Part model, mm, in its own coordinate system. Give positions to 0.01 mm unless a question says otherwise; leave off trailing zeros. Order: outer loops, then holes, each group sorted by start corner. A loop starts at its lowest first (then second) coordinate and runs counter-clockwise, first axis right, second up.
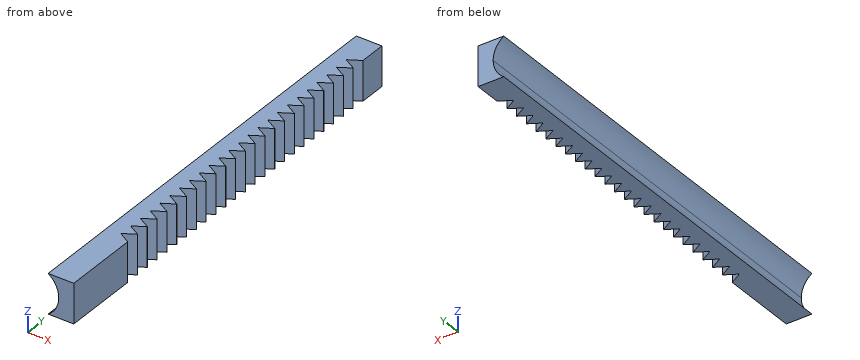
from build123d import *

# Parameters (mm, degrees)
BOSS_EXTRUDE1_DEPTH = 550
CUT_EXTRUDE1_DEPTH  = 73
BOSS_EXTRUDE2_DEPTH = 550


with BuildPart() as part:
    # Sketch1 → Boss-Extrude1 (new body)
    with BuildSketch(Plane(origin=(0, 0, 0), x_dir=(1, 0, 0), z_dir=(0, 1, 0))):
        with BuildLine():
            Line((43.301270189, -25), (69, -25))
            Line((69, -25), (69, 25))
            Line((69, 25), (43.301270189, 25))
            ThreePointArc((43.301270189, 25), (50, 0), (43.301270189, -25))
        make_face()
    extrude(amount=BOSS_EXTRUDE1_DEPTH)

    # Sketch2 → Cut-Extrude1 (cut)
    with BuildSketch(Plane.XY.offset(25)):
        Polygon((54, 489.993192311), (76.5, 477.002811254), (76.5, 502.983573367), align=None)
        Polygon((54, 507.493192311), (76.5, 494.502811254), (76.5, 520.483573367), align=None)
        Polygon((54, 472.493192311), (76.5, 459.502811254), (76.5, 485.483573367), align=None)
        Polygon((54, 454.993192311), (76.5, 442.002811254), (76.5, 467.983573367), align=None)
        Polygon((54, 437.493192311), (76.5, 424.502811254), (76.5, 450.483573367), align=None)
        Polygon((54, 419.993192311), (76.5, 407.002811254), (76.5, 432.983573367), align=None)
        Polygon((54, 402.493192311), (76.5, 389.502811254), (76.5, 415.483573367), align=None)
        Polygon((54, 384.993192311), (76.5, 372.002811254), (76.5, 397.983573367), align=None)
        Polygon((54, 367.493192311), (76.5, 354.502811254), (76.5, 380.483573367), align=None)
        Polygon((54, 349.993192311), (76.5, 337.002811254), (76.5, 362.983573367), align=None)
        Polygon((54, 332.493192311), (76.5, 319.502811254), (76.5, 345.483573367), align=None)
        Polygon((54, 314.993192311), (76.5, 302.002811254), (76.5, 327.983573367), align=None)
        Polygon((54, 297.493192311), (76.5, 284.502811254), (76.5, 310.483573367), align=None)
        Polygon((54, 279.993192311), (76.5, 267.002811254), (76.5, 292.983573367), align=None)
        Polygon((54, 262.493192311), (76.5, 249.502811254), (76.5, 275.483573367), align=None)
        Polygon((54, 244.993192311), (76.5, 232.002811254), (76.5, 257.983573367), align=None)
        Polygon((54, 227.493192311), (76.5, 214.502811254), (76.5, 240.483573367), align=None)
        Polygon((54, 209.993192311), (76.5, 197.002811254), (76.5, 222.983573367), align=None)
        Polygon((54, 192.493192311), (76.5, 179.502811254), (76.5, 205.483573367), align=None)
        Polygon((54, 174.993192311), (76.5, 162.002811254), (76.5, 187.983573367), align=None)
        Polygon((54, 157.493192311), (76.5, 144.502811254), (76.5, 170.483573367), align=None)
        Polygon((54, 139.993192311), (76.5, 127.002811254), (76.5, 152.983573367), align=None)
        Polygon((54, 122.493192311), (76.5, 109.502811254), (76.5, 135.483573367), align=None)
        Polygon((54, 104.993192311), (76.5, 92.002811254), (76.5, 117.983573367), align=None)
    extrude(amount=-CUT_EXTRUDE1_DEPTH, mode=Mode.SUBTRACT)

    # Sketch3 → Boss-Extrude2 (add)
    with BuildSketch(Plane(origin=(0, 550, 0), x_dir=(1, 0, 0), z_dir=(0, 1, 0))):
        with BuildLine():
            ThreePointArc((43.301270189, -25), (48.296291314, -12.940952255), (50, 0))
            ThreePointArc((50, 0), (46.433820369, -14.186371655), (36.583123952, -25))
            Line((36.583123952, -25), (43.301270189, -25))
        make_face()
        with BuildLine():
            ThreePointArc((50, 0), (48.296291314, 12.940952255), (43.301270189, 25))
            Line((43.301270189, 25), (36.583123952, 25))
            ThreePointArc((36.583123952, 25), (46.433820369, 14.186371655), (50, 0))
        make_face()
    extrude(amount=-BOSS_EXTRUDE2_DEPTH)


solid = part.part
Item 1: Band-saw the part on C-C on x = 63.5. Give the number of separate pieces and of enclosed holes in the cut face, plus the area to 3 significant figures.
Item 2: Drop flat-ended pins along their axis: P1, Ø8, axis at y = 111.5, z = -2, coming from the -X side; P2, Ø5, axis at y = 350.5, z = 8, coming from the -X side; P3, Ø12, axis at x = 59, y = 435, coming from the -Z side. Give the stop position or say it passes through.
Item 3: Band-saw the part on B-B on y = 45.5. List the corners of the cut face in (x, z), plus the area to 3 significant figures.
Item 4: Drill centre lines: probe 1 along Z at (x, y) = (40, 408); probe 2 along X at (y, z) = (499.5, -14.5); probe 3 along X at (y, z) = (494, 22). Where is each one in solid material? Low to high.
Item 5: Band-saw the part on A-A on x = 42. List the corners of the cut face in (y, z), plus the area to 3 significant figures.
Working result:
1. separate pieces: 25
1. enclosed holes: 0
1. area: 14,300 mm2
2. P1: stops at x = 49.39
2. P2: stops at x = 48.1
2. P3: stops at z = -25
3. outline: (36.58, -25) - (69, -25) - (69, 25) - (36.58, 25) arc R30 cw to start
3. area: 1,150 mm2
4. probe 1: z = -25 to -22.36, 22.36 to 25
4. probe 2: x = 46.26 to 67.84
4. probe 3: x = 40.4 to 60.94
5. outline: (0, -25) - (550, -25) - (550, -20.4) - (0, -20.4) - close; (0, 20.4) - (550, 20.4) - (550, 25) - (0, 25) - close
5. area: 5,060 mm2
